Autodesk Inventor part; units mm, degrees
ref_plane "YZ Plane" through (0, 0, 0) normal (1, 0, 0) x (0, 1, 0)
ref_plane "XZ Plane" through (0, 0, 0) normal (0, 1, 0) x (-1, 0, 0)
ref_plane "XY Plane" through (0, 0, 0) normal (0, 0, 1) x (1, 0, 0)
sketch "Sketch1" plane through (0, 0, 0) normal (1, 0, 0) x (0, 1, 0)
  circle A0 centre (0, 0) radius 20
  line L0 (-19.68, 3.5636) -> (-29, -47.9062)
  line L1 (19.68, 3.5636) -> (29, -47.9062)
  line L2 (11.5, 0) -> (-11.5, 0) construction
  line L3 (0, -48.5721) -> (0, 48.5721) construction
  arc A1 (-28.2326, -43.6683) -> (28.2326, -43.6683) centre (0, 0) ccw
  arc A2 (-29, -47.9062) -> (29, -47.9062) centre (0, 0) ccw
  point P0 (0, -56)
  point P1 (0, 0)
  dimension "d0" = 40
  dimension "d8" = 104
  dimension "d9" = 112
  dimension "d10" = 58
extrude "Extrusion1" add sketch "Sketch1" along normal blind 6
extrude "Extrusion2" add sketch "Sketch1" against normal blind 49 contours L1 A2 L0 A1
fillet "Fillet1" radius 10 1 edges at (0, 0, -52)
properties part number "thigh_connector"
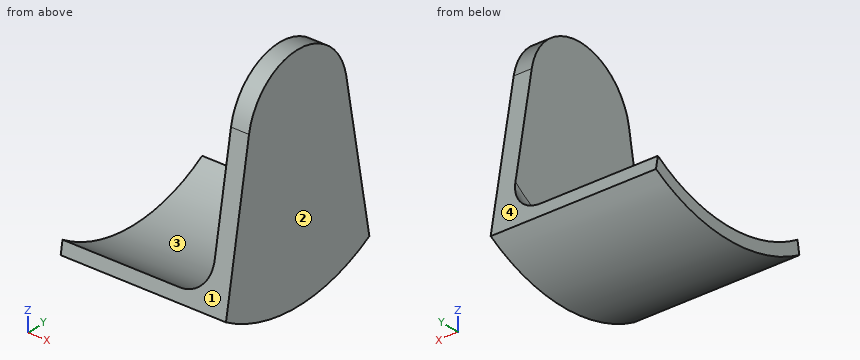
Input: part model. Units: mm. Frame: model coordinates. Face numbers are marked on the shaded views. Coordinates: 2 decimals unless noted, no trailing zeros. Loops run counter-clockwise (first coordinate to the right, second up) from the corner with the lowest first, then second, coordinate; pieces in that order, holes last. Notation, with made-up numbers: (-5.5, 4) - (36.5, 4) arc R12 ccw to (36.5, 26) - close; hole circle Ø4 at (41.25, 31.5). An arc over 180 degrees is marked (long way). Answer in a Markdown table with one row per item. Add a question column.
Item 1: Section query A-A on x = -24. Return the cut outline in (y, z), then the cut area to 3 significant figures.
Item 2: Mould query, pull axis Y, two halves, no side actions, for the marked faces 1, 2, 3 and 4. Classes: released by +Y, released by -Y, zero draft, split by the parting line, or undercut.
Item 3: Section query B-B on z = -17. Return the cut outline in (x, y), then the cut area to 3 significant figures.
Item 4: Line query: line 1 along X through (y, z) = (-7.5, -37.5); line 2 along Z through (x, y) = (-10, -16.5); line 3 along Z through (x, y) = (-16, 19.5). Output: solid intervals per line, ascending. Write a range as [from, to].
Item 5: Contact query for flat-ended pins moving along their axis: P1, Ø10, axis at x = -8.5, z = -12, coming from the -Y side; P2, Ø1, axis at y = 15.5, z = 12, coming from the -X side; P3, Ø12, axis at x = -2, y = -1.5, coming from the +Z side; P4, Ø2, axis at x = -18, y = -8, coming from the +Z side. Output: stop coordinate, or through.
Recorded:
| question | item | result |
|---|---|---|
| 1 | outline | (-29, -47.91) arc R56 ccw to (29, -47.91) - (28.23, -43.67) arc R52 cw to (-28.23, -43.67) - close |
| 1 | area | 241 mm^2 |
| 2 | face 1 | released by -Y |
| 2 | face 2 | zero draft |
| 2 | face 3 | undercut |
| 2 | face 4 | released by +Y |
| 3 | outline | (0, -23.4) - (6, -23.4) - (6, 23.4) - (0, 23.4) - close |
| 3 | area | 281 mm^2 |
| 4 | line 1 | [0, 6] |
| 4 | line 2 | [-53.51, -49.31] |
| 4 | line 3 | [-52.5, -48.21] |
| 5 | P1 | through |
| 5 | P2 | x = 0 |
| 5 | P3 | z = 20 |
| 5 | P4 | z = -51.22 |
